from build123d import *

# Parameters (mm, degrees)
F0_W      = 76.2
F0_H      = 76.2
F1_DEPTH  = 76.2
F2_W      = 25.4
F2_H      = 25.4
F3_DEPTH  = 12.7
F4_R      = 12.7
F5_DEPTH  = 12.7
F7_D      = 25.4
F9_DEPTH  = 38.1
F10_R     = 12.7
F11_DEPTH = 25.4


with BuildPart() as f1:
    # F0 (on Front) → F1 (new body)
    with BuildSketch(Plane.XZ):
        with Locations((-21.454936, 66.037557)):
            Rectangle(F0_W, F0_H)
    extrude(amount=F1_DEPTH)

    # F2 (on face) → F3 (join)
    with BuildSketch(Plane.XZ.offset(76.2)):
        with Locations((-22.974357, 63.60508)):
            Rectangle(F2_W, F2_H)
    extrude(amount=F3_DEPTH)

    # F4 (on face) → F5 (join)
    with BuildSketch(Plane.YZ.offset(16.645064)):
        with Locations((-34.295596, 82.468808)):
            Circle(F4_R)
    extrude(amount=F5_DEPTH)

    # F7 (through all)
    with Locations(Plane.XY.offset(104.137557)):
        with Locations((-10.916158, -49.894316)):
            Hole(F7_D / 2)

    # F8 (on face) → F9 (join)
    with BuildSketch(Plane(origin=(0, 0, 0), x_dir=(-1, 0, 0), z_dir=(0, 1, 0))):
        Polygon((13.244484, 97.82351), (22.827807, 74.300757), (38.407448, 94.361535), align=None)
    extrude(amount=F9_DEPTH)

    # F10 (on face) → F11 (join)
    with BuildSketch(Plane(origin=(-59.554936, 0, 0), x_dir=(0, -1, 0), z_dir=(-1, 0, 0))):
        with Locations((58.153983, 70.059642)):
            Circle(F10_R)
    extrude(amount=F11_DEPTH)


solid = f1.part
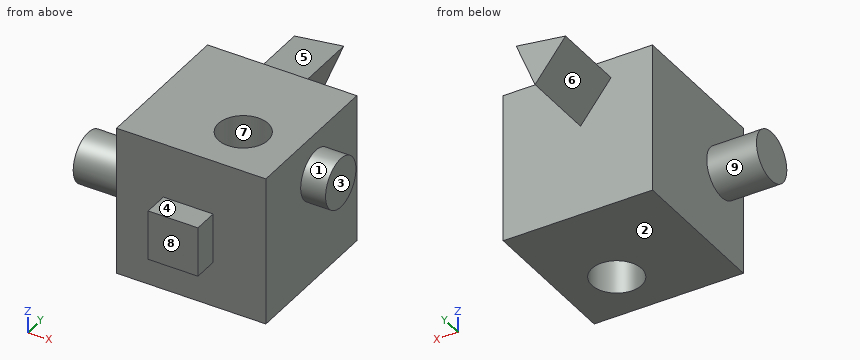
CAD build for the part. Positions are in the model's coordinates, mm. Face numbers are marked on the shaded views. A direction names the side the tool comes from. Round coordinates to 2 decimals unless told otherwise and drop trailing zeros. Write each loop counter-clockwise with the first axis right and the second up, starting at its lowest first coordinate (ties: lowest second). Pieces come first, ordered by that corner, then holes. Notation, with made-up numbers: M 1,59 L 8,59 A21 ccw 8,81 Z; hole C 82.5,15 d10. An arc over 180 degrees is marked long. Put each result on its own line as item: value. Start each with the question number.
1) Saw through at A-A, the plane x = -15. Write the cut outline in (y, z), and give its area (3 significant figures).
2) Pull direction Y, two halves, no side cores. Call the marked faces 6, 7, 8 and 9: pulls with the +Y half, pulls with the -Y half, needs draft (parallel to the pull), parting line crosses it, or undercut.
3) Pin check, flat tips, straight feed: pin 1 Ø23 at (x, z) = (-29, 62) entering from +Y; pin 2 Ø3 at (x, z) = (-4, 47.5) entering from -Y; pin 3 Ø6.5 at (y, z) = (-84, 61.5) entering from -X. Stop position of each tip, or through.
4) Drill centre lines: probe 1 along Y at (x, z) = (-10.5, 87.5); probe 2 along X at (y, z) = (-31, 80.5); probe 3 along X at (y, z) = (-75, 66). Where is each one in solid material? Low to high. Write a range as [from, to].
5) Saw through at D-D, the plane x = -30.5. Write the cut outline in (y, z), and give its area (3 significant figures).
6) Saw through at C-C, the plane y = 15. Write the cut outline in (x, z).
7) Saw through at B-B, the plane z = 53.5. Write the cut outline in (x, y).
8) 3-axis set-ups, long thin cutter, end or side, ignore diameter. For the marked faces 1, 2, 3, 4 and 5: which of +Z, -Z, +X, -X, +Y, -Y reach the whole face in a straight line?
Resolved:
1. outline: M -88.9,50.91 L -76.2,50.91 L -76.2,27.94 L -61.92,27.94 L -61.92,104.14 L -76.2,104.14 L -76.2,76.31 L -88.9,76.31 Z; M -37.87,27.94 L 0,27.94 L 0,93.51 L 38.1,93.51 L 38.1,97.58 L 0,97.58 L 0,104.14 L -37.87,104.14 Z
1. area: 4,450 mm²
2. face 6: needs draft
2. face 7: undercut
2. face 8: pulls with the -Y half
2. face 9: parting line crosses it
3. pin 1: y = 0
3. pin 2: y = -76.2
3. pin 3: x = -35.67
4. probe 1: [-76.2, -62.59], [-37.2, 0]
4. probe 2: [-59.55, 29.35]
4. probe 3: [-59.55, 16.65]
5. outline: M -88.9,50.91 L -76.2,50.91 L -76.2,27.94 L 0,27.94 L 0,84.18 L 38.1,84.18 L 38.1,95.45 L 0,95.45 L 0,104.14 L -76.2,104.14 L -76.2,76.31 L -88.9,76.31 Z
5. area: 6,560 mm²
6. outline: M -38.41,94.36 L -22.83,74.3 L -13.24,97.82 Z
7. outline: M -59.55,-76.2 L -35.67,-76.2 L -35.67,-88.9 L -10.27,-88.9 L -10.27,-76.2 L 16.65,-76.2 L 16.65,0 L -59.55,0 Z; hole C -10.92,-49.89 d25.4
8. face 1: +X
8. face 2: -Z, +X, -X, +Y, -Y
8. face 3: +Z, -Z, +X, +Y, -Y
8. face 4: +Z, +X, -X, -Y
8. face 5: +Z, -X, +Y
